```python
from build123d import *

# Parameters (mm, degrees)
SKETCH1_R           = 7
BOSS_EXTRUDE1_DEPTH = 12
SKETCH2_R           = 11.075
CUT_EXTRUDE1_DEPTH  = 8.5
SKETCH4_R           = 1.75
CUT_EXTRUDE4_DEPTH  = 13
SKETCH5_R           = 3.25
CUT_EXTRUDE5_DEPTH  = 3
SKETCH6_W           = 5.5
SKETCH6_H           = 12
BOSS_EXTRUDE2_DEPTH = 14
SKETCH7_R           = 2.75
CUT_EXTRUDE6_DEPTH  = 37.7
FILLET1_R           = 3


with BuildPart() as part:
    # Sketch1 → Boss-Extrude1 (new body)
    with BuildSketch(Plane(origin=(0, 0, 0), x_dir=(1, 0, 0), z_dir=(0, 1, 0))):
        with BuildLine():
            Line((-18.2, 15), (-18.2, 20))
            Line((-18.2, 20), (18.2, 20))
            Line((18.2, 20), (18.2, 15))
            Line((18.2, 15), (18.496206995, 0.374602179))
            ThreePointArc((18.496206995, 0.374602179), (0, -18.5), (-18.496206995, 0.374602179))
            Line((-18.496206995, 0.374602179), (-18.2, 15))
        make_face()
        Circle(SKETCH1_R, mode=Mode.SUBTRACT)
    extrude(amount=BOSS_EXTRUDE1_DEPTH)

    # Sketch2 → Cut-Extrude1 (cut)
    with BuildSketch(Plane.XZ):
        Circle(SKETCH2_R)
    extrude(amount=-CUT_EXTRUDE1_DEPTH, mode=Mode.SUBTRACT)

    # Sketch4 → Cut-Extrude4 (cut, through all)
    with BuildSketch(Plane.XZ):
        with Locations((10.253048327, 10.253048327)):
            Circle(SKETCH4_R)
        with Locations((10.253048327, -10.253048327)):
            Circle(SKETCH4_R)
        with Locations((-10.253048327, -10.253048327)):
            Circle(SKETCH4_R)
        with Locations((-10.253048327, 10.253048327)):
            Circle(SKETCH4_R)
    extrude(amount=-CUT_EXTRUDE4_DEPTH, mode=Mode.SUBTRACT)

    # Sketch5 → Cut-Extrude5 (cut)
    with BuildSketch(Plane(origin=(0, 12, 0), x_dir=(1, 0, 0), z_dir=(0, 1, 0))):
        with Locations((-10.253048327, 10.253048327)):
            Circle(SKETCH5_R)
        with Locations((10.253048327, 10.253048327)):
            Circle(SKETCH5_R)
        with Locations((10.253048327, -10.253048327)):
            Circle(SKETCH5_R)
        with Locations((-10.253048327, -10.253048327)):
            Circle(SKETCH5_R)
    extrude(amount=-CUT_EXTRUDE5_DEPTH, mode=Mode.SUBTRACT)

    # Sketch6 → Boss-Extrude2 (add)
    with BuildSketch(Plane(origin=(0, 0, -20), x_dir=(-1, 0, 0), z_dir=(0, 0, -1))):
        with Locations((-15.45, 6)):
            Rectangle(SKETCH6_W, SKETCH6_H)
        with Locations((15.45, 6)):
            Rectangle(SKETCH6_W, SKETCH6_H)
    extrude(amount=BOSS_EXTRUDE2_DEPTH)

    # Sketch7 → Cut-Extrude6 (cut, through all)
    with BuildSketch(Plane.ZY.offset(18.2)):
        with Locations((-28.501137854, 6)):
            Circle(SKETCH7_R)
    extrude(amount=-CUT_EXTRUDE6_DEPTH, mode=Mode.SUBTRACT)

    # Fillet1
    fillet1_edges = [part.edges().sort_by_distance(p)[0] for p in [
        (15.45, 0, -34),
        (15.45, 12, -34),
        (-15.45, 0, -34),
        (-15.45, 12, -34),
    ]]
    fillet(fillet1_edges, radius=FILLET1_R)


solid = part.part
```
Here's how the part is built. I have some questions about the finished solid (model axes, mm). A direction names the side the tool comes from. Give positions to 0.01 mm unless a question says otherwise; leave off trailing zeros. Loops run counter-clockwise (first coordinate to the right, second up) from the corner with the lowest first, then second, coordinate; pieces in that order, holes last. Notation, with made-up numbers: M 53.5,54 L 110.5,54 A14 ccw 110.5,61 Z; hole C 37,84.5 d7. An arc over 180 degrees is marked long. Use one line per item in the form item = value. Start each with the question number.
Q1. If we section it at A-A (x = 0): Write out the boundary of the cut face in (y, z) (3 decimals).
Q2. Thinking about a two-plate mould opening in X: for faces 4 (the cylindrical face through (-2.4, 4.19, -10.81)), 5 (the cylindrical face through (-15.49, 11.14, -33.1)), 6 (the flat face through (-18.2, 6, -24)), which applies, +X half, -X half, draft (parallel to the pull), parting line (faces both ways), or undercut?
Q3. If we section it at D-D (z = -4.5): Write out the boundary of the cut face in (x, y), then the cut area to 3 significant figures.
Q4. If we section it at B-B (y = 5): Write out the boundary of the cut face in (x, z) (3 decimals), then the cut area to 3 significant figures.
Q5. Will these pins go through, and if not, where does the flat tip stop? pin 1 Ø2 at (y, z) = (10, -21) entering from +X; pin 2 Ø3 at (x, z) = (-9, -9.5) entering from +Y; pin 3 Ø18 at (x, z) = (0, 0) entering from -Y.
Q6. If we section it at C-C (z = -28): Write out the boundary of the cut face in (x, y).
Q7. I need wall thicknesses on line 1 along X through (y, z) = (10, -29); line 2 along X through (y, z) = (7.5, -10); line 3 along X through (y, z) = (9, -18). Which ranges of each line are inside material? Lowest first, please.
Q8. Which directions (+Z, -Z, +X, -X, +Y, -Y) give clear straight access to the entire face, cutting with the end or side of a thin tool? Please do faces 1 (the flat face through (-0.2, 8.5, -7.2)), 2 (the cylindrical face through (-8.584, 4.437, 10.779)), 3 (the cylindrical face through (9.83, 10.521, -13.475)).
Taken from the geometry:
q1.outline = M 0,-20 L 12,-20 L 12,-7 L 8.5,-7 L 8.5,-11.075 L 0,-11.075 Z; M 0,11.075 L 8.5,11.075 L 8.5,7 L 12,7 L 12,18.5 L 0,18.5 Z
q2.face_4 = undercut
q2.face_5 = draft
q2.face_6 = -X half
q3.outline = M -18.41,0 L -10.12,0 L -10.12,8.5 L -5.36,8.5 L -5.36,12 L -18.41,12 Z; M 5.36,8.5 L 10.12,8.5 L 10.12,0 L 18.41,0 L 18.41,12 L 5.36,12 Z
q3.area = 232 mm^2
q4.outline = M -18.496,-0.375 L -18.2,-15 L -18.2,-25.939 L -12.7,-25.939 L -12.7,-20 L 12.7,-20 L 12.7,-25.939 L 18.2,-25.939 L 18.2,-15 L 18.496,-0.375 A18.5 ccw long Z; M -18.2,-34 L -12.7,-34 L -12.7,-31.063 L -18.2,-31.063 Z; M 12.7,-34 L 18.2,-34 L 18.2,-31.063 L 12.7,-31.063 Z; hole C -10.253,-10.253 d3.5; hole C -10.253,10.253 d3.5; hole C 0,0 d22.15; hole C 10.253,-10.253 d3.5; hole C 10.253,10.253 d3.5
q4.area = 944 mm^2
q5.pin_1 = 18.2
q5.pin_2 = 9
q5.pin_3 = 8.5
q6.outline = M -18.2,0 L -12.7,0 L -12.7,3.3 L -18.2,3.3 Z; M -18.2,8.7 L -12.7,8.7 L -12.7,12 L -18.2,12 Z; M 12.7,0 L 18.2,0 L 18.2,3.3 L 12.7,3.3 Z; M 12.7,8.7 L 18.2,8.7 L 18.2,12 L 12.7,12 Z
q7.line_1 = -18.2 to -12.7, 12.7 to 18.2
q7.line_2 = -18.3 to -11.98, -8.52 to -4.76, 4.76 to 8.52, 11.98 to 18.3
q7.line_3 = -18.2 to 18.2
q8.face_1 = -Y
q8.face_2 = +Y, -Y
q8.face_3 = +Y
